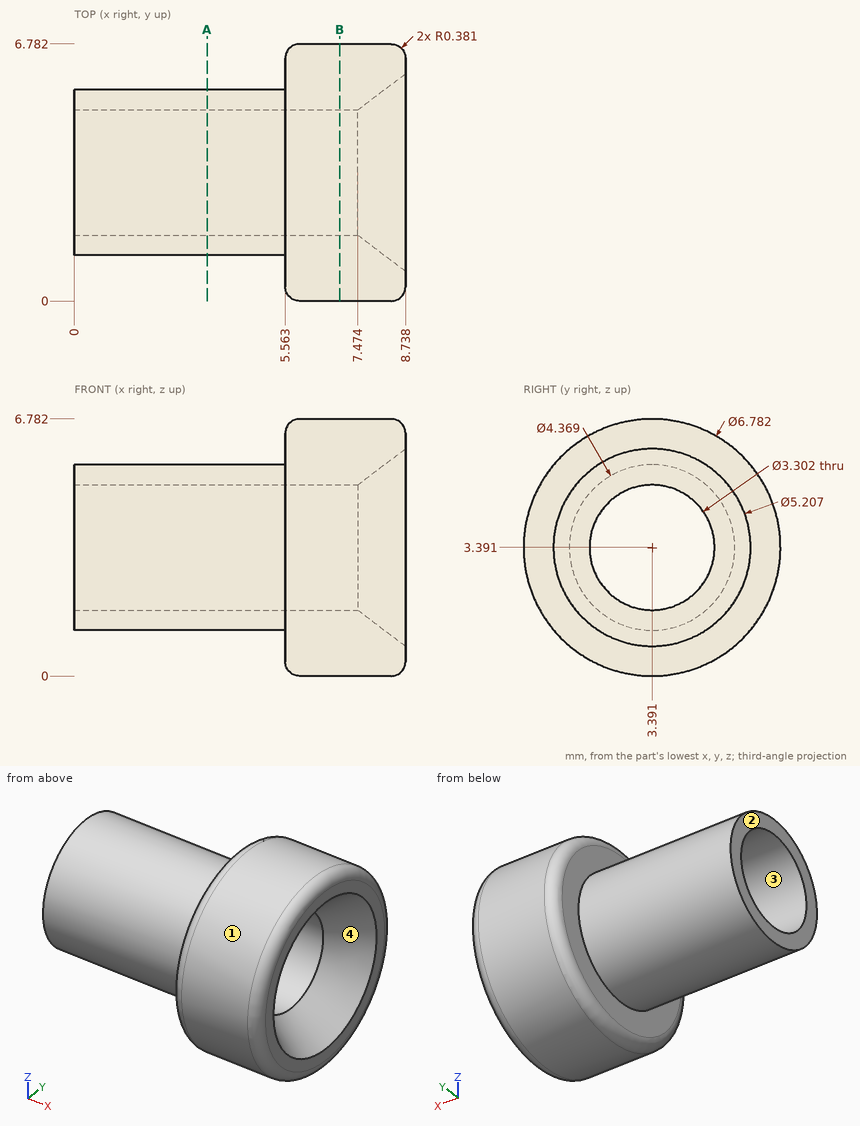
Geometry: see drawing. Coordinates: mm, zero at the bounding-box minimum. Round coordinates to 2 decimals unless told otherwise and drop trailing zeros. Loops run counter-clockwise (first coordinate to the right, second up) from the corner with the lowest first, then second, coordinate; pieces in that order, holes last. Notation, with made-up numbers: M 30,35 L 87,35 A24 cw 87,54 Z; hole C 19.5,26.25 d9. An arc over 180 degrees is marked long. Use a Markdown table: item, result. Add a question column.
1. Line query: line 1 (Z direction, x = 6.5, y = 2) (1 decimal); line 2 (X direction, y = 5.5, z = 1.25); line 3 (Y direction, x = 8.25, z = 4.25) (1 decimal). Output: solid intervals per line, ascending.
2. Section query B-B on x = 7. Return the cut outline in (y, z).
3. Section query A-A on x = 3.5. Return the cut outline in (y, z) (1 decimal).
4. Contact query for flat-ended pins moving along their axis: P1, Ø3, axis at x = 1.5, y = 3, coming from the +Z side (1 decimal); P2, Ø1.5, axis at x = 2.5, z = 1.5, coming from the +Y side. Output: stop coordinate, or through.
5. Mould query, pull axis Z, two halves, no side actions, for the marked faces 1, 2, 3 and 4. Classes: pulls with the +Z half, pulls with the -Z half, needs draft (parallel to the pull), parting line crosses it, or undercut.
Reported:
| question | item | result |
|---|---|---|
| 1 | line 1 | z = 0.3 to 2.5, 4.3 to 6.5 |
| 1 | line 2 | x = 5.56 to 8.74 |
| 1 | line 3 | y = 0.1 to 1.3, 5.5 to 6.7 |
| 2 | outline | C 3.39,3.39 d6.78; hole C 3.39,3.39 d3.3 |
| 3 | outline | C 3.4,3.4 d4.4; hole C 3.4,3.4 d3.3 |
| 4 | P1 | stops at z = 5.6 |
| 4 | P2 | stops at y = 5.25 |
| 5 | face 1 | parting line crosses it |
| 5 | face 2 | needs draft |
| 5 | face 3 | undercut |
| 5 | face 4 | undercut |
